Could you check a few things on this drawing? It's one solid part, dimensions in mm from its lowest x, y, z. A direction names the side the tool comes from. Give positions to 0.01 mm unless a question says otherwise; leave off trailing zeros. Loops run counter-clockwise (first coordinate to the right, second up) from the corner with the lowest first, then second, coordinate; pieces in that order, holes last.
Q1. For the marked faces 4, 5 and 6, which set-ups out of +Z, -Z, +X, -X, +Y, -Y let a thin tool reach every point of the face, with its end or its side?
Q2. Suppose I cut it at C-C (z = 32). List the corners of the cut face in (x, y) for me, and give its area (3 significant figures).
Q3. Suppose I cut it at D-D (y = 26). List the corners of the cut face in (x, z) for me, and give its area (3 significant figures).
Q4. Suppose I cut it at B-B (y = 11). List the corners of the cut face in (x, z) for me.
Q5. I need wall thicknesses on probe 1 along Y at (x, z) = (81.5, 66.5) (3 decimals); probe 2 along X at (y, z) = (31, 88); probe 3 along X at (y, z) = (82, 14.5). Which ranges of each line are inside material? Lowest first, please.
Q6. Thinking about a two-plate mould opening in Y: for the marked faces 1, 2 and 3, which applies, pulls with the +Y half, pulls with the -Y half, needs draft (parallel to the pull), parting line crosses it, or undercut?
Q7. Suppose I cut it at A-A (x = 43). List the corners of the cut face in (y, z) for me (3 decimals), and give its area (3 significant figures).
Q8. I'm going to push flat-ended pins straight in: P1, Ø9.5, axis at x = 5.5, y = 40, coming from the +Z side; P2, Ø3, axis at x = 64.5, z = 71, coming from the +Y side (3 decimals); P3, Ø10, axis at x = 80, y = 26.5, coming from the -Z side. Where does each tip first touch, or does it pass through?
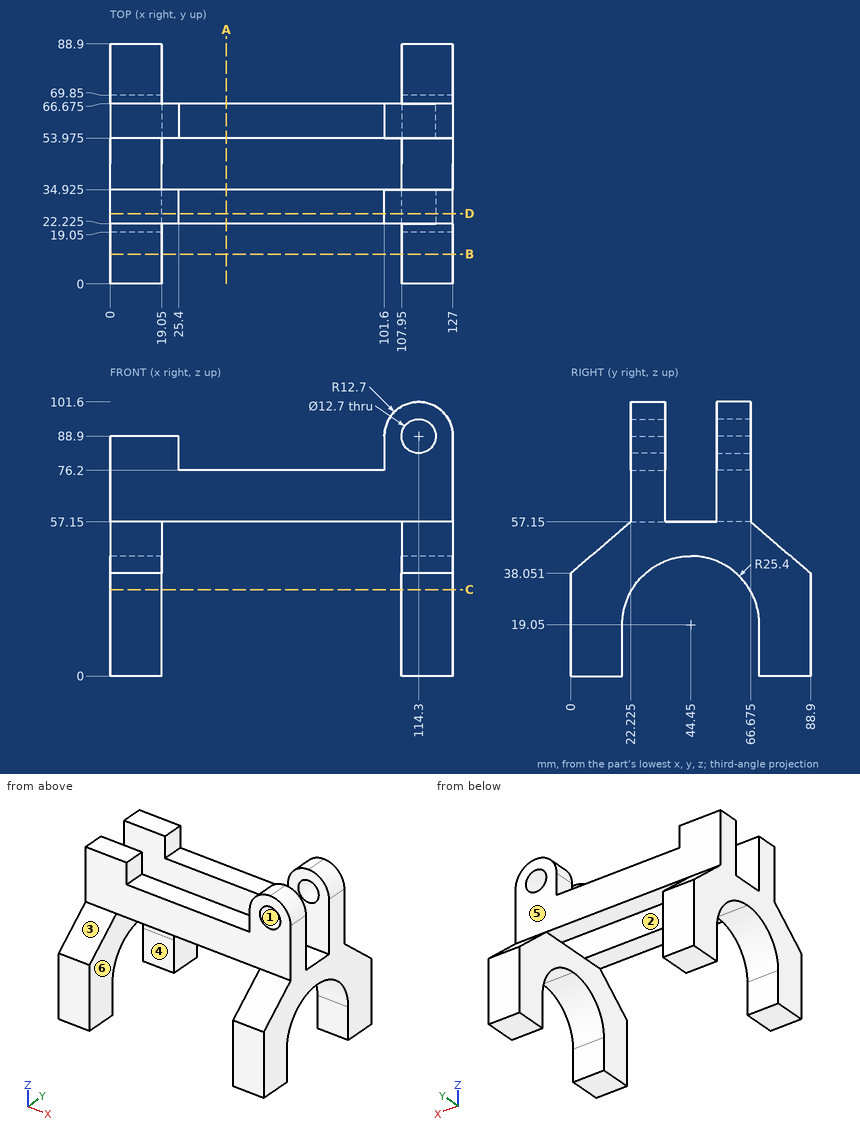
Solutions:
1. face 4: -Z, +X, -X
1. face 5: +Z, +X, -X, +Y
1. face 6: -Z, +Y, -Y
2. outline: (0, 0) - (19.05, 0) - (19.05, 22.6) - (0, 22.6) - close; (0, 66.3) - (19.05, 66.3) - (19.05, 88.9) - (0, 88.9) - close; (107.95, 0) - (127, 0) - (127, 22.6) - (107.95, 22.6) - close; (107.95, 66.3) - (127, 66.3) - (127, 88.9) - (107.95, 88.9) - close
2. area: 1,720 mm2
3. outline: (0, 36.51) - (19.05, 36.51) - (19.05, 57.15) - (107.95, 57.15) - (107.95, 36.51) - (127, 36.51) - (127, 88.9) arc R12.7 ccw to (101.6, 88.9) - (101.6, 76.2) - (25.4, 76.2) - (25.4, 88.9) - (0, 88.9) - close; hole circle Ø12.7 at (114.3, 88.9)
3. area: 3,980 mm2
4. outline: (0, 0) - (19.05, 0) - (19.05, 47.5) - (0, 47.5) - close; (107.95, 0) - (127, 0) - (127, 47.5) - (107.95, 47.5) - close
5. probe 1: y = 22.225 to 34.925, 53.975 to 66.675
5. probe 2: x = 0 to 25.4, 101.6 to 108.01, 120.59 to 127
5. probe 3: x = 0 to 19.05, 107.95 to 127
6. face 1: needs draft
6. face 2: undercut
6. face 3: pulls with the -Y half
7. outline: (22.225, 57.15) - (34.925, 57.15) - (34.925, 76.2) - (22.225, 76.2) - close; (53.975, 57.15) - (66.675, 57.15) - (66.675, 76.2) - (53.975, 76.2) - close
7. area: 484 mm2
8. P1: stops at z = 57.15
8. P2: stops at y = 66.675
8. P3: stops at z = 57.15
